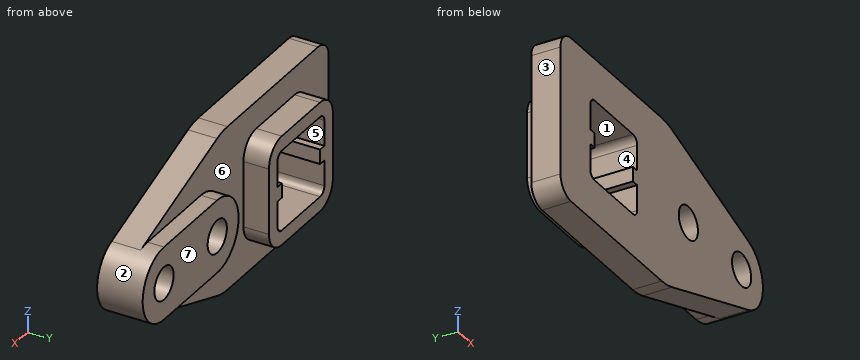
from build123d import *

# Parameters (mm, degrees)
SKETCH_1_W          = 100
SKETCH_1_H          = 90
EXTRUDE_1_DEPTH     = 16
FILLET_1_R          = 10
SKETCH_4_W          = 60
SKETCH_4_H          = 60
EXTRUDE_2_DEPTH     = 30
FILLET_3_R          = 12
CUT_EXTRUDE_1_DEPTH = 46
FILLET_4_R          = 4
EXTRUDE_4_DEPTH     = 16
SKETCH_10_R         = 9
EXTRUDE_5_DEPTH     = 25
FILLET_6_R          = 30


with BuildPart() as part:
    # 草图1 → 凸台-拉伸1 (new body)
    with BuildSketch(Plane(origin=(0, 0, 0), x_dir=(1, 0, 0), z_dir=(0, 1, 0))):
        with Locations((50, 0)):
            Rectangle(SKETCH_1_W, SKETCH_1_H)
    extrude(amount=EXTRUDE_1_DEPTH)

    # 圆角1
    fillet_1_edges = [part.edges().sort_by_distance(p)[0] for p in [
        (0, 8, -45),
        (0, 8, 45),
    ]]
    fillet(fillet_1_edges, radius=FILLET_1_R)

    # 草图4 → 凸台-拉伸2 (add)
    with BuildSketch(Plane(origin=(0, 0, 0), x_dir=(1, 0, 0), z_dir=(0, 1, 0))):
        with Locations((50, 0)):
            Rectangle(SKETCH_4_W, SKETCH_4_H)
    extrude(amount=EXTRUDE_2_DEPTH)

    # 圆角3
    fillet_3_edges = [part.edges().sort_by_distance(p)[0] for p in [
        (20, 23, -30),
        (20, 23, 30),
        (80, 23, 30),
        (80, 23, -30),
    ]]
    fillet(fillet_3_edges, radius=FILLET_3_R)

    # 草图5 → 切除-拉伸1 (cut)
    with BuildSketch(Plane(origin=(0, 0, 0), x_dir=(1, 0, 0), z_dir=(0, 1, 0))):
        Polygon((28, -4), (28, -22), (72, -22), (72, -4), (68, -4), (68, 4), (72, 4), (72, 22), (28, 22), (28, 4), (32, 4), (32, -4), align=None)
    extrude(amount=CUT_EXTRUDE_1_DEPTH, mode=Mode.SUBTRACT)

    # 圆角4
    fillet_4_edges = [part.edges().sort_by_distance(p)[0] for p in [
        (28, 15, -22),
        (28, 15, 22),
        (72, 15, 22),
        (72, 15, -22),
    ]]
    fillet(fillet_4_edges, radius=FILLET_4_R)

    # 草图9 → 凸台-拉伸4 (add)
    with BuildSketch(Plane(origin=(0, 0, 0), x_dir=(1, 0, 0), z_dir=(0, 1, 0))):
        with BuildLine():
            ThreePointArc((100, 1e-09), (105.857864376, 14.142135624), (120, 20))
            Line((120, 20), (168.98254652, 19.974102944))
            ThreePointArc((168.98254652, 19.974102944), (170.010573991, 19.999997205), (171.038573506, 19.973015923))
            ThreePointArc((171.038573506, 19.973015923), (173.782842055, 19.638994526), (176.45483392, 18.929741653))
            Line((176.45483392, 18.929741653), (100, 45))
            Line((100, 45), (100, 1e-09))
        make_face()
        with BuildLine():
            ThreePointArc((120, -20), (105.857864376, -14.142135623), (100, 1e-09))
            Line((100, 1e-09), (100, -45))
            Line((100, -45), (176.45483392, -18.929741653))
            ThreePointArc((176.45483392, -18.929741653), (173.271480317, -19.730621291), (170, -20))
            Line((170, -20), (120, -20))
        make_face()
    extrude(amount=EXTRUDE_4_DEPTH)

    # 草图10 → 凸台-拉伸5 (add)
    with BuildSketch(Plane(origin=(0, 0, 0), x_dir=(1, 0, 0), z_dir=(0, 1, 0))):
        with BuildLine():
            Line((120, 20), (170, 20))
            ThreePointArc((170, 20), (190, 0), (170, -20))
            Line((170, -20), (120, -20))
            ThreePointArc((120, -20), (100, 0), (120, 20))
        make_face()
        with Locations(Location((120, 0, 0), (0, 0, 270))):
            Circle(SKETCH_10_R, mode=Mode.SUBTRACT)
        with Locations(Location((170, 0, 0), (0, 0, 270))):
            Circle(SKETCH_10_R, mode=Mode.SUBTRACT)
    extrude(amount=EXTRUDE_5_DEPTH)

    # 圆角6
    fillet_6_edges = [part.edges().sort_by_distance(p)[0] for p in [
        (100, 8, -45),
        (100, 8, 45),
    ]]
    fillet(fillet_6_edges, radius=FILLET_6_R)


solid = part.part
Can you work these out from the model? Positions are in its coordinate system, mm. Face numbers are marked on the shaded views. A direction names the side the tool comes from. Give positions to 0.01 mm unless a question says otherwise; leave off trailing zeros. Write each loop counter-clockwise with the first axis right and the second up, starting at its lowest first coordinate (ties: lowest second). Pieces come first, ordered by that corner, then holes. Notation, with made-up numbers: M -17.75,12 L 4.25,12 A22 ccw 4.25,19 Z; hole C -17.5,-12 d8. An arc over 180 degrees is marked long. Answer in a Markdown table with one row per item. Add a question column.
Item 1: Please list where these lines run through material, in increasing order: L1, parallel to X at y = 9.25, z = 0; L2, parallel to X at y = 18.5, z = 0; L3, parallel to X at y = 28.5, z = 7.
Item 2: We'd pull the mould along X, two halves only. Please class the marked faces 1, 2, 3 and 4: released by +X, released by -X, zero draft, split by the parting line, or undercut.
Item 3: Imagine slicing it at B-B, the plane z = 0. Write out the boundary of the cut face in (x, y).
Item 4: Imagine slicing it at A-A, the plane y = 21. State how many separate pieces and enclosed holes the cut face has, plus the area to 3 significant figures.
Item 5: On a 3-axis mill with a long thin cutter (end or side, diameter ignored), from which of +Z, -Z, +X, -X, +Y, -Y can I reach the whole of each face in a straight line? I mean the marked faces 5, 6 and 7. Say none if no direction works.
Item 6: For pin 1 Ø15.5 at (x, y) = (52, 20) entering from +Z; pin 2 Ø4 at (x, y) = (158.5, 23.5) entering from +Z; pin 3 Ø12 at (y, z) = (11.5, -14) entering from +X; pin 4 Ø2.5 at (x, y) = (142, 22) entering from -Z, each with a flat end and sliding along its axis, tell me the tip position at first contact or that it passes through.
Item 7: Imagine slicing it at D-D, the plane z = -12. Write out the boundary of the cut face in (x, y).
Item 8: Imagine slicing it at C-C, the plane y = 11.25. Write out the boundary of the cut face in (x, z).
Evaluation:
| question | item | result |
|---|---|---|
| 1 | L1 | x = 0 to 32, 68 to 111, 129 to 161, 179 to 190 |
| 1 | L2 | x = 20 to 32, 68 to 80, 100 to 111, 129 to 161, 179 to 190 |
| 1 | L3 | x = 20 to 28, 72 to 80 |
| 2 | face 1 | undercut |
| 2 | face 2 | released by +X |
| 2 | face 3 | released by -X |
| 2 | face 4 | undercut |
| 3 | outline | M 0,0 L 32,0 L 32,30 L 20,30 L 20,16 L 0,16 Z; M 68,0 L 111,0 L 111,25 L 100,25 L 100,16 L 80,16 L 80,30 L 68,30 Z; M 129,0 L 161,0 L 161,25 L 129,25 Z; M 179,0 L 190,0 L 190,25 L 179,25 Z |
| 4 | separate pieces | 2 |
| 4 | enclosed holes | 3 |
| 4 | area | 4,370 mm² |
| 5 | face 5 | +Y, -Y |
| 5 | face 6 | +Y |
| 5 | face 7 | +Z, -Z, +X, +Y |
| 6 | pin 1 | stops at z = 45 |
| 6 | pin 2 | stops at z = 20 |
| 6 | pin 3 | stops at x = 188.33 |
| 6 | pin 4 | stops at z = -20 |
| 7 | outline | M 0,0 L 28,0 L 28,30 L 20,30 L 20,16 L 0,16 Z; M 72,0 L 186,0 L 186,25 L 104,25 L 104,16 L 80,16 L 80,30 L 72,30 Z |
| 8 | outline | M 0,-35 A10 ccw 10,-45 L 95.03,-45 A30 ccw 104.71,-43.39 L 176.45,-18.93 A20 ccw 176.45,18.93 L 104.71,43.39 A30 ccw 95.03,45 L 10,45 A10 ccw 0,35 Z; hole M 28,-18 A4 ccw 32,-22 L 68,-22 A4 ccw 72,-18 L 72,-4 L 68,-4 L 68,4 L 72,4 L 72,18 A4 ccw 68,22 L 32,22 A4 ccw 28,18 L 28,4 L 32,4 L 32,-4 L 28,-4 Z; hole C 120,0 d18; hole C 170,0 d18 |
